Can you work these out from the drawing? Everything is in mm from the part's minimum corner. Give positions to 0.01 mm unless a question says otherwise; leave off trailing zeros. Order: outer loops, then holes, each group sorted by start corner. A loop starts at its lowest first (then second) coordinate and runs counter-clockwise, first axis right, second up. Notation, with made-up numbers: M 85,43 L 110,43 A16 cw 110,73 Z; hole C 18,69.5 d2. An arc over 180 degrees is marked long. Answer as a JSON object with one key per item and string values.
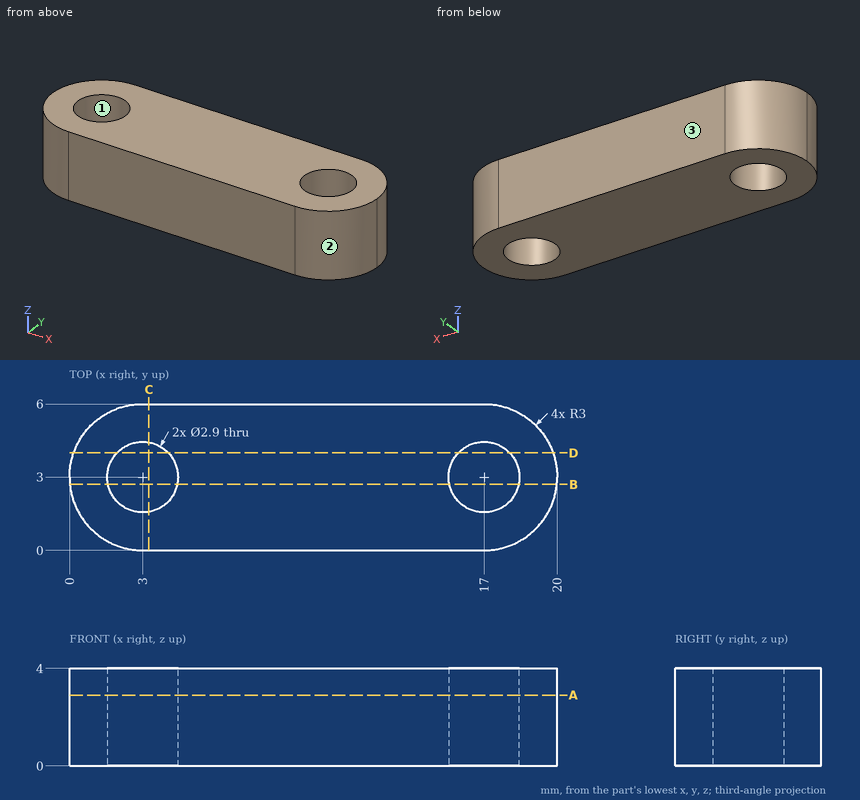
1) I need wall thicknesses on L1, parallel to X at y = 3, z = 2.8; L2, parallel to X at y = 3.6, z = 2.1; L3, parallel to Y at x = 17, z = 1.25. Which ranges of each line are inside material? Lowest first, please.
Results found:
{"L1": "x = 0 to 1.55, 4.45 to 15.55, 18.45 to 20", "L2": "x = 0.06 to 1.68, 4.32 to 15.68, 18.32 to 19.94", "L3": "y = 0 to 1.55, 4.45 to 6"}
2) I want a section at B-B on y = 2.7. Write out the boundary of the cut face in (x, z) (1 decimal), and give its area (3 significant figures).
Results found:
{"outline": "M 0,0 L 1.6,0 L 1.6,4 L 0,4 Z; M 4.4,0 L 15.6,0 L 15.6,4 L 4.4,4 Z; M 18.4,0 L 20,0 L 20,4 L 18.4,4 Z", "area": "57.2 mm²"}
3) I want a section at C-C on x = 3.25. Write out the boundary of the cut face in (y, z).
Results found:
{"outline": "M 0,0 L 1.57,0 L 1.57,4 L 0,4 Z; M 4.43,0 L 6,0 L 6,4 L 4.43,4 Z"}
4) I want a section at A-A on z = 2.9. Count the separate pieces of the cut face and the enclosed holes in it, and give its area (3 significant figures).
Results found:
{"separate pieces": "1", "enclosed holes": "2", "area": "99.1 mm²"}
5) I want a section at D-D on y = 4. Write out the boundary of the cut face in (x, z).
Results found:
{"outline": "M 0.17,0 L 1.95,0 L 1.95,4 L 0.17,4 Z; M 4.05,0 L 15.95,0 L 15.95,4 L 4.05,4 Z; M 18.05,0 L 19.83,0 L 19.83,4 L 18.05,4 Z"}
6) I'm going to push flat-ended pins straight in: pin 1 Ø2 at (x, z) = (7, 2.5) entering from -Y; pin 2 Ø1 at (y, z) = (4, 2) entering from +X. Where does each tip first touch, or does it pass through?
Results found:
{"pin 1": "stops at y = 0", "pin 2": "stops at x = 19.96"}
7) Thinking about a two-plate mould opening in X: for the marked faces 1, 2 and 3, which applies, pulls with the +X half, pulls with the -X half, needs draft (parallel to the pull), parting line crosses it, or undercut?
Results found:
{"face 1": "undercut", "face 2": "pulls with the +X half", "face 3": "needs draft"}
